```python
from build123d import *

# Parameters (mm, degrees)
SKETCH2_W                    = 210.920124673
SKETCH2_H                    = 90.17
BASE_FLANGE1_DEPTH           = 0.635
EDGE_FLANGE1_STRIP_W         = 3.81
EDGE_FLANGE1_STRIP_H         = 0.635
EDGE_FLANGE1_STRIP_CUT_DEPTH = 210.920124673
EDGE_FLANGE1_DEPTH           = 210.920124673
EDGE_FLANGE4_DEPTH           = 36.83
EDGE_FLANGE7_START           = -89.535
EDGE_FLANGE7_DEPTH           = 19.685
EDGE_FLANGE8_DEPTH           = 210.920124673
CUT_EXTRUDE1_REACH           = 235.927
SKETCH41_W                   = 31.449187445
SKETCH41_H                   = 25.469780901


# Read off the part's stored shape, not the designer's step: Edge-Flange7
# Sheet-metal steps are written as plain solids
with BuildPart() as part:
    # Sketch2 → Base-Flange1 (new body)
    with BuildSketch(Plane(origin=(0, 0, 0), x_dir=(1, 0, 0), z_dir=(0, 1, 0))):
        with Locations((105.460062337, 45.085)):
            Rectangle(SKETCH2_W, SKETCH2_H)
    extrude(amount=-BASE_FLANGE1_DEPTH)

    # Edge-Flange1 strip (across the edge) → Edge-Flange1 strip cut (cut)
    with BuildSketch(Plane(origin=(0, -0.635, -90.17), x_dir=(0, 0, 1), z_dir=(1, 0, 0))):
        with Locations((-1.27, -0.3175)):
            Rectangle(EDGE_FLANGE1_STRIP_W, EDGE_FLANGE1_STRIP_H)
    extrude(amount=EDGE_FLANGE1_STRIP_CUT_DEPTH, mode=Mode.SUBTRACT)

    # Edge-Flange1 section (across the edge) → Edge-Flange1 (add)
    with BuildSketch(Plane(origin=(0, -0.635, -90.17), x_dir=(0, 0, 1), z_dir=(1, 0, 0))):
        with BuildLine():
            Line((-0.635, 0.635), (-0.635, 37.465))
            Line((-0.635, 37.465), (0, 37.465))
            Line((0, 37.465), (0, 0.635))
            ThreePointArc((0, 0.635), (0.185987194, 0.185987194), (0.635, 0))
            Line((0.635, 0), (0.635, -0.635))
            ThreePointArc((0.635, -0.635), (-0.263025612, -0.263025612), (-0.635, 0.635))
        make_face()
    extrude(amount=EDGE_FLANGE1_DEPTH)

    # Edge-Flange4 section (across the edge) → Edge-Flange4 (add)
    with BuildSketch(Plane(origin=(211.555124673, -38.1, -90.17), x_dir=(-1, 0, 0), z_dir=(0, 1, 0))):
        with BuildLine():
            Line((-0.635, 0.635), (-0.635, 20.32))
            Line((-0.635, 20.32), (0, 20.32))
            Line((0, 20.32), (0, 0.635))
            ThreePointArc((0, 0.635), (0.185987194, 0.185987194), (0.635, 0))
            Line((0.635, 0), (0.635, -0.635))
            ThreePointArc((0.635, -0.635), (-0.263025612, -0.263025612), (-0.635, 0.635))
        make_face()
    edge_flange4 = extrude(amount=EDGE_FLANGE4_DEPTH)

    # Edge-Flange7 outline → Edge-Flange7 (add)
    with BuildSketch(Plane.XY.offset(EDGE_FLANGE7_START)):
        with BuildLine():
            ThreePointArc((212.190124673, -0.508), (211.818150285, 0.390025612), (210.920124673, 0.762))
            Line((210.920124673, 0.762), (188.995937227, 0.762))
            Line((188.995937227, 0.762), (188.995937227, 0.127))
            Line((188.995937227, 0.127), (210.920124673, 0.127))
            ThreePointArc((210.920124673, 0.127), (211.369137479, -0.058987194), (211.555124673, -0.508))
            Line((211.555124673, -0.508), (211.555124673, -1.27))
            Line((211.555124673, -1.27), (212.190124673, -1.27))
            Line((212.190124673, -1.27), (212.190124673, -0.508))
        make_face()
    edge_flange7 = extrude(amount=EDGE_FLANGE7_DEPTH)

    # Mirror1: Edge-Flange4, Edge-Flange7 across plane
    add(edge_flange4.mirror(Plane.ZY.offset(-105.460062336)))
    add(edge_flange7.mirror(Plane.ZY.offset(-105.460062336)))

    # Edge-Flange8 section (across the edge) → Edge-Flange8 (add)
    with BuildSketch(Plane(origin=(210.920124673, -0.635, 0.635), x_dir=(0, 0, -1), z_dir=(-1, 0, 0))):
        with BuildLine():
            Line((-0.635, 0.635), (-0.635, 5.715))
            Line((-0.635, 5.715), (0, 5.715))
            Line((0, 5.715), (0, 0.635))
            ThreePointArc((0, 0.635), (0.185987194, 0.185987194), (0.635, 0))
            Line((0.635, 0), (0.635, -0.635))
            ThreePointArc((0.635, -0.635), (-0.263025612, -0.263025612), (-0.635, 0.635))
        make_face()
    extrude(amount=EDGE_FLANGE8_DEPTH)

    # Sketch41 → Cut-Extrude1 (cut, up to next)
    with BuildSketch(Plane(origin=(0, 0, 0), x_dir=(1, 0, 0), z_dir=(0, 1, 0)), mode=Mode.PRIVATE) as cut_extrude1_sk1:
        with Locations((41.124593723, 10.12510955)):
            Rectangle(SKETCH41_W, SKETCH41_H)
    cut_extrude1_tool1 = extrude(cut_extrude1_sk1.sketch, amount=-CUT_EXTRUDE1_REACH, mode=Mode.PRIVATE) & part.part
    add(cut_extrude1_tool1.solids().sort_by_distance((41.124594, 0, -10.12511))[0], mode=Mode.SUBTRACT)


solid = part.part
```
Geometry check sheet. Reference: the model listing, model coordinates, mm. A direction names the side the tool comes from. Give positions to 0.01 mm unless a question says otherwise; leave off trailing zeros. Loops run counter-clockwise (first coordinate to the right, second up) from the corner with the lowest first, then second, coordinate; pieces in that order, holes last. Notation, with made-up numbers: (-22.5, -5.5) - (7.5, -5.5) arc R15 ccw to (7.5, 19.5) - close; hole circle Ø8 at (-28.75, 82.5). An arc over 180 degrees is marked (long way). Use CSV: the item, a comma, the result in double quotes. Start each with the question number.
Q1. Go/stop test with flat-tipped pins: pin 1 Ø10 at (x, z) = (11.5, -81) entering from -Y (3 decimals); pin 2 Ø7 at (y, z) = (-2, -8) entering from +X; pin 3 Ø1.4 at (x, z) = (-1, -90) entering from +Y. Record where each tip stops, or that it passes through.
Q2. Access from +Z, -Z, +X, -X, +Y, -Y to the whole of each face (thin tool, end or side, straight path). Record for faces 1 (the face through (211.555, -19, -80)), 2 (the face through (135, -4, 0.635)), 3 (the face through (104, -0.635, -45)), 4 (the face through (25.4, -0.3, -8.1)).
Q3. Section check A-A, the plane y = -3.5. Record the cut outline in (x, z) (3 decimals), and give its area (3 significant figures).
Q4. Scan lines: probe 1 along X at (y, z) = (-17.5, -73) (3 decimals); probe 2 along Z at (x, y) = (167, -3) (3 decimals); probe 3 along Z at (x, y) = (49, -10) (3 decimals). Record each from-to range of solid material in increasing order. Write a range as from..to.
Q5. Section check D-D, the plane x = 182.5. Record the cut outline in (y, z) (3 decimals), and give its area (3 significant figures).
Q6. Section check B-B, the plane x = 13.5. Record the cut outline in (y, z) (3 decimals).
Q7. Section check C-C, the plane z = -6. Record the cut outline in (x, y) (3 decimals).
Findings below:
1,pin 1,"stops at y = -0.635"
1,pin 2,"stops at x = 210.92"
1,pin 3,"stops at y = 0.67"
2,face 1,"+Z, -Y"
2,face 2,"+X, -X, -Y"
2,face 3,"-Y"
2,face 4,"+Z, +Y, -Y"
3,outline,"(-1.27, -89.535) arc R1.27 ccw to (0, -90.805) - (210.92, -90.805) arc R1.27 ccw to (212.19, -89.535) - (212.19, -69.85) - (211.555, -69.85) - (211.555, -89.535) arc R0.635 cw to (210.92, -90.17) - (0, -90.17) arc R0.635 cw to (-0.635, -89.535) - (-0.635, -69.85) - (-1.27, -69.85) - close; (0, 0.635) - (25.4, 0.635) - (25.4, 1.27) - (0, 1.27) - close; (56.849, 0.635) - (210.92, 0.635) - (210.92, 1.27) - (56.849, 1.27) - close"
3,area,"275 mm^2"
4,probe 1,"x = -1.27..-0.635, 211.555..212.19"
4,probe 2,"z = -90.805..-90.17, 0.635..1.27"
4,probe 3,"z = -90.805..-90.17"
5,outline,"(-38.1, -90.805) - (-1.27, -90.805) arc R1.27 ccw to (0, -89.535) - (0, 0) arc R1.27 ccw to (-1.27, 1.27) - (-6.35, 1.27) - (-6.35, 0.635) - (-1.27, 0.635) arc R0.635 cw to (-0.635, 0) - (-0.635, -89.535) arc R0.635 cw to (-1.27, -90.17) - (-38.1, -90.17) - close"
5,area,"85.4 mm^2"
6,outline,"(-38.1, -90.805) - (-1.27, -90.805) arc R1.27 ccw to (0, -89.535) - (0, 0) arc R1.27 ccw to (-1.27, 1.27) - (-6.35, 1.27) - (-6.35, 0.635) - (-1.27, 0.635) arc R0.635 cw to (-0.635, 0) - (-0.635, -89.535) arc R0.635 cw to (-1.27, -90.17) - (-38.1, -90.17) - close; (0.127, -89.535) - (0.762, -89.535) - (0.762, -69.85) - (0.127, -69.85) - close"
7,outline,"(0, -0.635) - (25.4, -0.635) - (25.4, 0) - (0, 0) - close; (56.849, -0.635) - (210.92, -0.635) - (210.92, 0) - (56.849, 0) - close"
